The figure shows three views and two pictorial views of one solid part (mm, origin at its lowest corner). Answer the questions. A direction names the side the tool comes from. Give positions to 0.01 mm unless a question says otherwise; leave off trailing zeros. Write each loop counter-clockwise with the first axis right and the second up, starting at its lowest first coordinate (ties: lowest second). Pieces come first, ordered by that corner, then holes. Notation, with made-up numbers: M -37,47 L -16,47 A8 ccw -16,57 Z; hole C 44,42 d2. An arc over 180 degrees is marked long. Return JSON: item names as keys, results as strings.
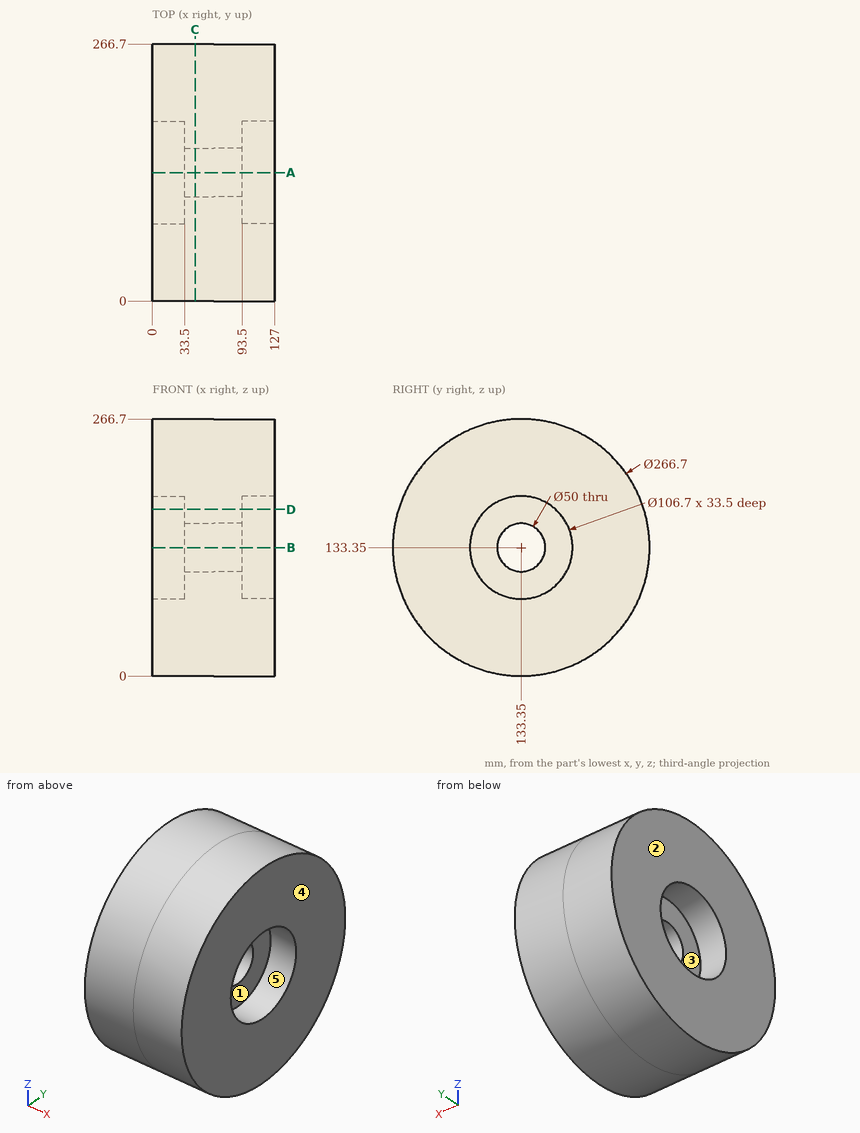
Item 1: Find the intervals of material crossed by line 1 (Z direction, x = 15.5, y = 133.35); line 2 (Z direction, x = 84.25, y = 133.35), in increasing order.
Geometry results:
{"line 1": "z = 0 to 80, 186.7 to 266.7", "line 2": "z = 0 to 108.35, 158.35 to 266.7"}
Item 2: Given pin 1 Ø3 at (x, y) = (44, 64.5) entering from +Z; pin 2 Ø4 at (x, z) = (104, 36) entering from +Y; pin 3 Ø8 at (x, y) = (74.5, 159.5) entering from -Z, each flat-ended and moving along its own axis, determine where each tip first touches the part or whether it passes through.
Geometry results:
{"pin 1": "stops at z = 248.44", "pin 2": "stops at y = 226.57", "pin 3": "stops at z = 1.85"}
Item 3: A cutting plane is placed at C-C, the plane x = 44.5. Write down the section's boundary in (y, z).
Geometry results:
{"outline": "C 133.35,133.35 d266.7; hole C 133.35,133.35 d50"}
Item 4: A cutting plane is placed at A-A, the plane y = 133.35. Write down the section's boundary in (x, z), plus the area to 3 significant figures.
Geometry results:
{"outline": "M 0,0 L 127,0 L 127,80 L 93.5,80 L 93.5,108.35 L 33.5,108.35 L 33.5,80 L 0,80 Z; M 0,186.7 L 33.5,186.7 L 33.5,158.35 L 93.5,158.35 L 93.5,186.7 L 127,186.7 L 127,266.7 L 0,266.7 Z", "area": "23,700 mm2"}
Item 5: Which of the six approach directions +Z, -Z, +X, -X, +Y, -Y give full straight-line access (tool end or side, diameter ignored) to the marked faces 3, 4 and 5?
Geometry results:
{"face 3": "-X", "face 4": "+Z, -Z, +X, +Y, -Y", "face 5": "+X"}
Item 6: A cutting plane is placed at D-D, the plane z = 173. Write down the section's boundary in (x, y), plus the area to 3 significant figures.
Geometry results:
{"outline": "M 0,6.03 L 127,6.03 L 127,97.66 L 93.5,97.66 L 93.5,169.04 L 127,169.04 L 127,260.67 L 0,260.67 L 0,169.04 L 33.5,169.04 L 33.5,97.66 L 0,97.66 Z", "area": "27,600 mm2"}
Item 7: Determine the mould class of the marked faces 1 and 2 for opening direction Y: +Y half, -Y half, draft (parallel to the pull), parting line (faces both ways), or undercut.
Geometry results:
{"face 1": "undercut", "face 2": "draft"}
